Could you check a few things on this model? Use its own coordinates, in mm. A direction names the side the tool comes from. Give positions to 0.01 mm unless a question says otherwise; leave off trailing zeros. Loops run counter-clockwise (first coordinate to the right, second up) from the corner with the lowest first, then second, coordinate; pieces in that order, holes last. Notation, with made-up numbers: (60.5, 80.25) - (79.5, 80.25) arc R22 ccw to (79.5, 93.25) - close; hole circle Ø6 at (-13.5, 13.25). An arc over 180 degrees is marked (long way). Write each question's results on one line, items separated by ' | '. Start each with the question number.
1) I want a section at A-A, the plane z = 12.5. Write out the boundary of the cut face in (x, y), and give its area (3 significant figures).
2) I want a section at B-B, the plane x = 0. Write out the boundary of the cut face in (y, z), and give its area (3 significant figures).
3) If we mould it in two halves opening along X, with no side actions, what happens to faces 1 (the face through (7.88, -21.47, -12.54)), 2 (the face through (-72.008, -2, 12)), 3 (the face through (72.008, -2, 12))? For each: +X half, -X half, draft (parallel to the pull), parting line (faces both ways), or undercut.
4) I want a section at C-C, the plane y = -10. Write out the boundary of the cut face in (x, z), and give its area (3 significant figures).
5) On a 3-axis mill with a long thin cutter (end or side, diameter ignored), from which of +Z, -Z, +X, -X, +Y, -Y can I reach the whole of each face in a straight line? I mean faces 4 (the face through (0, -3.728, 13)), 5 (the face through (-17, -38.728, -8)). Say none if no direction works.
6) If I drill on probe 1 along X at (y, z) = (-31, 12.5); probe 2 along Z at (x, y) = (3, -7); probe 3 along Z at (x, y) = (-8.5, -20.5), over which ranges is the centre line in solid material (lowest first)? Write a range as [from, to].
from build123d import *

# Parameters (mm, degrees)
SKETCH1_W           = 41.147295424
SKETCH1_H           = 21.419140084
BOSS_EXTRUDE1_DEPTH = 25
SKETCH2_R           = 7.5
CUT_EXTRUDE1_DEPTH  = 10
SCALE1_SCALE        = 3.5


with BuildPart() as part:
    # Sketch1 → Boss-Extrude1 (new body)
    with BuildSketch(Plane.XY):
        Rectangle(SKETCH1_W, SKETCH1_H)
    extrude(amount=BOSS_EXTRUDE1_DEPTH)

    # Sketch2 → Cut-Extrude1 (cut)
    with BuildSketch(Plane.XZ.offset(10.709570042)):
        with Locations(Location((0, 12.5, 0), (0, 0, 270))):
            Circle(SKETCH2_R)
    extrude(amount=-CUT_EXTRUDE1_DEPTH, mode=Mode.SUBTRACT)


with BuildPart() as part_1:
    # Scale1: scaled about (0, 0.497852103, 12.5)
    add(part.part.scale(SCALE1_SCALE).moved(Location((0, -1.244630257, -31.25))))


solid = part_1.part
Answers:
1) outline: (-72.01, -38.73) - (-26.25, -38.73) - (-26.25, -3.73) - (26.25, -3.73) - (26.25, -38.73) - (72.01, -38.73) - (72.01, 36.24) - (-72.01, 36.24) - close | area: 8,960 mm2
2) outline: (-38.73, -31.25) - (36.24, -31.25) - (36.24, 56.25) - (-38.73, 56.25) - (-38.73, 38.75) - (-3.73, 38.75) - (-3.73, -13.75) - (-38.73, -13.75) - close | area: 4,720 mm2
3) face 1: undercut | face 2: -X half | face 3: +X half
4) outline: (-72.01, -31.25) - (72.01, -31.25) - (72.01, 56.25) - (-72.01, 56.25) - close; hole circle Ø52.5 at (0, 12.5) | area: 10,400 mm2
5) face 4: -Y | face 5: +Z, -Z, +X, -X, -Y
6) probe 1: x = [-72.01, -26.25], [26.25, 72.01] | probe 2: z = [-31.25, -13.58], [38.58, 56.25] | probe 3: z = [-31.25, -12.34], [37.34, 56.25]
